Geometry: final body of the model. Coordinates: model frame, mm. Face numbers are marked on the shaded views. A direction names the side the tool comes from. Give positions to 0.01 mm unless a question says otherwise; leave off trailing zeros. Order: outer loops, then holes, each group sorted by start corner. A loop starts at its lowest first (then second) coordinate and runs counter-clockwise, first axis right, second up. Notation, with made-up numbers: (41, 7) - (98, 7) arc R24 cw to (98, 41) - close; hole circle Ø9 at (21.25, 83). An arc over 180 degrees is marked (long way). Put each result on its own line as item: value. Start each with the question number.
1. Ray query, line 1 along Y through (x, z) = (-10, 0.75); line 2 along Z through (x, y) = (-6.5, -5.5); line 3 along Y through (x, z) = (45.5, -17.5). Return the intervals inside material, ascending. Write a range as from..to.
2. Section A-A on x = -10. Return the cut outline in (y, z).
3. First-contact query: P1, Ø22.5, axis at x = 28.5, y = 6.5, coming from the -Z side; P2, Ø1.1, axis at y = -15, z = 0.5, coming from the +X side. Flat tips, straight axial feed; report the tip coordinate or a pass-through.
4. Section C-C on z = -30.5. Return the cut outline in (x, y), plus the area to 3 significant figures.
5. Set-up query: the marked faces 1 and 2. Return all of +Z, -Z, +X, -X, +Y, -Y with unobstructed straight access to the full face (end or side cutting, diameter ignored); none if empty.
6. Section B-B on x = 9.5. Return the cut outline in (y, z), plus the area to 3 significant figures.
7. Section D-D on y = -30.5. Return the cut outline in (x, z).
from build123d import *

# Parameters (mm, degrees)
BOSS_EXTRUDE1_DEPTH = 1
SKETCH4_R           = 1.5
CUT_EXTRUDE5_DEPTH  = 1
SKETCH5_R           = 5
BOSS_EXTRUDE2_DEPTH = 40


with BuildPart() as part:
    # Sketch1 → Boss-Extrude1 (new body)
    with BuildSketch(Plane.XY):
        Polygon((-20, 35), (-20, -40), (0, -40), (0, 0), (15, 15), (55, 15), (55, 35), align=None)
    extrude(amount=BOSS_EXTRUDE1_DEPTH)

    # Sketch4 → Cut-Extrude5 (cut)
    with BuildSketch(Plane.XY.offset(1)):
        with Locations((-10, 25.000149563)):
            Circle(SKETCH4_R)
    extrude(amount=-CUT_EXTRUDE5_DEPTH, mode=Mode.SUBTRACT)

    # Sketch5 → Boss-Extrude2 (add)
    with BuildSketch(Plane.XY.offset(1)):
        with Locations((43.007008147, 25)):
            Circle(SKETCH5_R)
    extrude(amount=-BOSS_EXTRUDE2_DEPTH)


solid = part.part
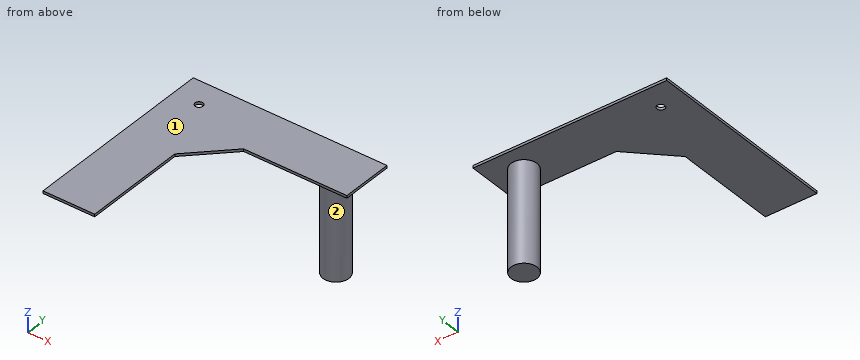
Resolved:
1. line 1: -40..23.5, 26.5..35
1. line 2: 0..1
1. line 3: 20.67..29.33
2. outline: (-40, 0) - (23.5, 0) - (23.5, 1) - (-40, 1) - close; (26.5, 0) - (35, 0) - (35, 1) - (26.5, 1) - close
3. P1: z = 0
3. P2: x = 0
4. outline: circle Ø10 at (43.01, 25)
4. area: 78.5 mm^2
5. face 1: +Z, +X, -X, +Y, -Y
5. face 2: -Z
6. outline: (9.5, 0) - (35, 0) - (35, 1) - (9.5, 1) - close
6. area: 25.5 mm^2
7. outline: (-20, 0) - (0, 0) - (0, 1) - (-20, 1) - close
